```python
from build123d import *

# Parameters (mm, degrees)
BOX001_W     = 80
BOX001_H     = 80
BOX001_DEPTH = 40


with BuildPart() as obj1:
    # Sphere → Sphere (revolve)
    with BuildSketch(Plane(origin=(38, 38, 0), x_dir=(1, 0, 0), z_dir=(0, -1, 0))):
        with BuildLine():
            ThreePointArc((0, -38), (38, 0), (0, 38))
            Line((0, 38), (0, -38))
        make_face()
    revolve(axis=Axis((38, 38, 0), (0, 0, 1)))


with BuildPart() as obj2:
    # Box001 → Box001 (new body)
    with BuildSketch(Plane(origin=(-2, -2, 0), x_dir=(1, 0, 0), z_dir=(0, 0, 1))):
        with Locations((40, 40)):
            Rectangle(BOX001_W, BOX001_H)
    extrude(amount=BOX001_DEPTH)


with BuildPart() as fusion003:
    # Sphere002 → Sphere002 (revolve)
    with BuildSketch(Plane(origin=(38, 38, -42), x_dir=(1, 0, 0), z_dir=(0, -1, 0))):
        with BuildLine():
            ThreePointArc((0, -12), (12, 0), (0, 12))
            Line((0, 12), (0, -12))
        make_face()
    revolve(axis=Axis((38, 38, -42), (0, 0, 1)))

    # Fusion003: union obj1, obj2
    add(obj1.part)
    add(obj2.part)


with BuildPart() as dome:
    # Sphere001 → Sphere001 (revolve)
    with BuildSketch(Plane(origin=(38, 38, 0), x_dir=(1, 0, 0), z_dir=(0, -1, 0))):
        with BuildLine():
            ThreePointArc((0, -40), (40, 0), (0, 40))
            Line((0, 40), (0, -40))
        make_face()
    revolve(axis=Axis((38, 38, 0), (0, 0, 1)))

    # Cut: cut Fusion003
    add(fusion003.part, mode=Mode.SUBTRACT)


with BuildPart() as dome_1:
    # Cut placement: moved
    add(dome.part.moved(Location((0, 2, 1))))


solid = dome_1.part
```
Input: part model. Units: mm. Frame: model coordinates. Give positions to 0.01 mm unless a question says otherwise; leave off trailing zeros. Order: outer loops, then holes, each group sorted by start corner. A loop starts at its lowest first (then second) coordinate and runs counter-clockwise, first axis right, second up. Notation, with made-up numbers: M 20.5,15.5 L 35.5,15.5 A28 ccw 35.5,42.5 Z; hole C 76,60.25 d6. An arc over 180 degrees is marked long. One line per question, with ' | ' between items. Start each with the question number.
1. Section query A-A (x = 43.5). Return the cut outline in (y, z).
2. Section query B-B (y = 48). Return the cut outline in (x, z).
3. Material intervals for probe 1 along X at (y, z) = (27, -17.5); probe 2 along Y at (x, z) = (56.5, -25.5); probe 3 along X at (y, z) = (64.5, -25), sorted ascending. Write a range as [from, to].
4. Section query D-D (x = 22.5). Return the cut outline in (y, z).
5. Section query C-C (z = -25). Return the cut outline in (x, y).
6. First-contact query: pin 1 Ø8 at (x, z) = (59.5, -26.5) entering from -Y; pin 2 Ø2 at (x, z) = (15, -8.5) entering from +Y; pin 3 Ø8 at (x, y) = (39, 16.5) entering from +Z. Flat tips, straight axial feed; report the tip coordinate or a pass-through.
Here are the results:
1) outline: M 0.38,1 A39.62 ccw 29.98,-37.33 A10.67 cw 30.88,-35.48 A37.6 cw 2.4,1 Z; M 49.12,-35.48 A10.67 cw 50.02,-37.33 A39.62 ccw 79.62,1 L 77.6,1 A37.6 cw Z
2) outline: M -1.19,1 A39.19 ccw 29.84,-37.33 A8.94 cw 30.97,-35.48 A37.15 cw 0.85,1 Z; M 45.03,-35.48 A8.94 cw 46.16,-37.33 A39.19 ccw 77.19,1 L 75.15,1 A37.15 cw Z
3) probe 1: [5, 7.46], [68.54, 71] | probe 2: [16.43, 20.01], [59.99, 63.57] | probe 3: [20.01, 25.05], [50.95, 55.99]
4) outline: M 3.13,1 A36.87 ccw 76.87,1 L 74.7,1 A34.7 cw 5.3,1 Z
5) outline: C 38,40 d60.79; hole C 38,40 d55.43
6) pin 1: y = 14.61 | pin 2: y = 72.09 | pin 3: z = -25.2
